Part model, mm, in its own coordinate system. A direction names the side the tool comes from. Round coordinates to 2 decimals unless told otherwise and drop trailing zeros. One line per question, with ' | ' between items. Start each with the question number.
1) Wall check: probe 1 along Z at (x, y) = (0, 7.8); probe 2 along X at (y, z) = (8.25, 33); probe 3 along Z at (x, y) = (-0.25, -7). Give the ranges that are in metal, low to high. Write a range as [from, to].
2) Tool access for faces 5 (the face through (0, 0, 32)), 6 (the face through (1.5, 3.6, 10.1)), 7 (the face through (0.89, 7.92, 8.89)), 8 (the face through (0, 2.1, 2)): list every direction of +Z, -Z, +X, -X, +Y, -Y with a clear straight run to the whole face (end or side of a thin tool).
3) Drop flat-ended pins along their axis: pin 1 Ø1.4 at (x, y) = (0.5, 0.5) entering from -Z; pin 2 Ø3 at (x, z) = (-8.5, 8.5) entering from +Y; pin 3 Ø5.5 at (x, z) = (-0.5, 8.5) entering from -Y. Give the stop position or say it passes through.
4) Mould opens along Z. For faces 1 (the face through (0, -10.5, 34)), 2 (the face through (2, 2.1, 8)), 3 (the face through (0, 0, 15)), 4 (the face through (1.5, 3.6, 4.9)) say: pulls with the +Z half, pulls with the -Z half, needs draft (parallel to the pull), parting line crosses it, or undercut.
```python
from build123d import *

# Parameters (mm, degrees)
SKETCH1_R           = 10
BOSS_EXTRUDE1_DEPTH = 30
SKETCH2_W           = 27.4
SKETCH2_H           = 27.4
BOSS_EXTRUDE2_DEPTH = 5
SKETCH3_W           = 21
SKETCH3_H           = 21
CUT_EXTRUDE1_DEPTH  = 3
SKETCH7_W           = 47.139349652
SKETCH7_H           = 47.139349652
SKETCH7_W_2         = 27.4
SKETCH7_H_2         = 27.4
CUT_EXTRUDE2_DEPTH  = 78
CUT_EXTRUDE3_DEPTH  = 15
CUT_EXTRUDE4_DEPTH  = 3
SKETCH11_R          = 1.65
CUT_EXTRUDE5_DEPTH  = 12


with BuildPart() as part:
    # Sketch1 → Boss-Extrude1 (new body)
    with BuildSketch(Plane.XY):
        Circle(SKETCH1_R)
    extrude(amount=BOSS_EXTRUDE1_DEPTH)

    # Sketch2 → Boss-Extrude2 (add)
    with BuildSketch(Plane.XY.offset(30)):
        Rectangle(SKETCH2_W, SKETCH2_H)
    extrude(amount=BOSS_EXTRUDE2_DEPTH)

    # Sketch3 → Cut-Extrude1 (cut)
    with BuildSketch(Plane.XY.offset(35)):
        Rectangle(SKETCH3_W, SKETCH3_H)
    extrude(amount=-CUT_EXTRUDE1_DEPTH, mode=Mode.SUBTRACT)

    # Sketch6 → Revolve1 (revolve)
    with BuildSketch(Plane(origin=(0, 0, 0), x_dir=(0, 0, -1), z_dir=(1, 0, 0))):
        with BuildLine():
            Line((-30, 0), (-30, 20))
            add(Edge.make_bspline(
                [(-30, 20), (-22.099947356, 11.248565128), (-4.613209845, 10), (0, 10)],
                knots=[0, 0, 0, 0, 1, 1, 1, 1], degree=3))
            Line((0, 10), (0, 0))
            Line((0, 0), (-30, 0))
        make_face()
    revolve(axis=Axis((0, 0, 63.541170981), (0, 0, 1)))

    # Sketch7 → Cut-Extrude2 (cut)
    with BuildSketch(Plane.XY.offset(30)):
        Rectangle(SKETCH7_W, SKETCH7_H)
        Rectangle(SKETCH7_W_2, SKETCH7_H_2, mode=Mode.SUBTRACT)
    extrude(amount=-CUT_EXTRUDE2_DEPTH, mode=Mode.SUBTRACT)

    # Sketch8 → Cut-Extrude3 (cut)
    with BuildSketch(Plane(origin=(0, 0, 0), x_dir=(-1, 0, 0), z_dir=(0, 0, -1))):
        with BuildLine():
            Line((-1.616322988, 2.1), (1.616322988, 2.1))
            ThreePointArc((1.616322988, 2.1), (0, -2.65), (-1.616322988, 2.1))
        make_face()
    extrude(amount=-CUT_EXTRUDE3_DEPTH, mode=Mode.SUBTRACT)

    # Sketch10 → Cut-Extrude4 (cut)
    with BuildSketch(Plane.XZ.offset(-2.1)):
        Polygon((0, 4.035898385), (3, 5.767949192), (3, 9.232050808), (0, 10.964101615), (-15.10195651, 10.964101615), (-15.10195651, 4.035898385), align=None)
    extrude(amount=-CUT_EXTRUDE4_DEPTH, mode=Mode.SUBTRACT)

    # Sketch11 → Cut-Extrude5 (cut)
    with BuildSketch(Plane.XZ.offset(-5.1)):
        with Locations((0, 7.5)):
            Circle(SKETCH11_R)
    extrude(amount=-CUT_EXTRUDE5_DEPTH, mode=Mode.SUBTRACT)


solid = part.part
```
Answer key:
1) probe 1: z = [0, 5.85], [9.15, 32] | probe 2: x = [-13.7, -10.5], [10.5, 13.7] | probe 3: z = [0, 32]
2) face 5: +Z | face 6: -X | face 7: +Y | face 8: -Z
3) pin 1: stops at z = 15 | pin 2: stops at y = 8.14 | pin 3: stops at y = -11.17
4) face 1: needs draft | face 2: undercut | face 3: pulls with the -Z half | face 4: undercut
